```python
from build123d import *

# Parameters (mm, degrees)
SKETCH_2_R          = 1.5
CUT_EXTRUDE_1_DEPTH = 19.493242009


with BuildPart() as part:
    # 草图1 → 旋转1 (revolve)
    with BuildSketch(Plane.XY, mode=Mode.PRIVATE) as revolve_1_sk:
        Polygon((4, 0), (4, 15.5), (5, 15.5), (5, 5.5), (11, 5.5), (11, 2), (5, 2), (5, 0), align=None)
    revolve(revolve_1_sk.sketch.rotate(Axis((0, -4.166666667, 0), (0, 1, 0)), 90), axis=Axis((0, -4.166666667, 0), (0, 1, 0)))

    # 草图2 → 切除-拉伸1 (cut, through all)
    with BuildSketch(Plane(origin=(0, 5.5, 0), x_dir=(1, 0, 0), z_dir=(0, 1, 0))):
        with Locations(Location((0, 8, 0), (0, 0, 270))):
            Circle(SKETCH_2_R)
        with Locations(Location((8, 0, 0), (0, 0, 270))):
            Circle(SKETCH_2_R)
        with Locations(Location((0, -8, 0), (0, 0, 270))):
            Circle(SKETCH_2_R)
        with Locations(Location((-8, 0, 0), (0, 0, 270))):
            Circle(SKETCH_2_R)
    extrude(amount=-CUT_EXTRUDE_1_DEPTH, mode=Mode.SUBTRACT)


solid = part.part
```
Geometry: final body of the model. Coordinates: model frame, mm. A direction names the side the tool comes from. Round coordinates to 2 decimals unless told otherwise and drop trailing zeros. Write each loop counter-clockwise with the first axis right and the second up, starting at its lowest first coordinate (ties: lowest second). Pieces come first, ordered by that corner, then holes. Notation, with made-up numbers: (64, 73.25) -> (90, 73.25) arc R19 ccw to (90, 90.25) -> close; hole circle Ø10 at (13, -16). An arc over 180 degrees is marked (long way). Use CSV: the item, a comma, the result in double quotes. Start each with the question number.
Q1. Pull-direction query (X, two-part tool) for faces 4 (the face through (2, 5.5, 5)), 5 (the face through (0.07, 3.77, -9.5)), 6 (the face through (10.74, 3.73, 2.38)); classes: pulls with the +X half, pulls with the -X half, needs draft (parallel to the pull), parting line crosses it, or undercut.
Q2. Section C-C (y = 4.5). Return loops of the section in (x, z), plus the area to 3 significant figures.
Q3. Section B-B (x = 0). Return loops of the section in (y, z).
Q4. First-contact query: pin 1 Ø1.8 at (x, z) = (0, -8) entering from -Y; pin 2 Ø5 at (x, z) = (-8, 0) entering from +Y; pin 3 Ø6 at (y, z) = (5, 4) entering from +X; pin 4 Ø4 at (x, z) = (8, -5) entering from -Y. Flat tips, straight axial feed; report the tip coordinate or a pass-through.
Q5. Reachability of faces 1 (the face through (5, 2, -2)), 2 (the face through (6.536, 3.774, -0.325)), 3 (the face through (0, 10, 5)) from +Z, -Z, +X, -X, +Y, -Y: full face, straight path, thin tool, end or side. Return the list, or none.
Q6. Section A-A (z = 0). Return loops of the section in (x, y), plus the area to 3 significant figures.
Q7. Section D-D (z = -7.5). Return loops of the section in (x, y), plus the area to 3 significant figures.
Q8. Line query: L1, parallel to X at y = 3.1, z = 0; L2, parallel to Y at x = 2.75, z = 4.5; L3, parallel to Z at x = -3, y = 4. Output: solid intervals per line, ascending.
Result sheet:
1,face 4,"needs draft"
1,face 5,"undercut"
1,face 6,"parting line crosses it"
2,outline,"circle Ø22 at (0, 0); hole circle Ø3 at (-8, 0); hole circle Ø8 at (0, 0); hole circle Ø3 at (0, -8); hole circle Ø3 at (0, 8); hole circle Ø3 at (8, 0)"
2,area,"302 mm²"
3,outline,"(0, -5) -> (2, -5) -> (2, -6.5) -> (5.5, -6.5) -> (5.5, -5) -> (15.5, -5) -> (15.5, -4) -> (0, -4) -> close; (0, 4) -> (15.5, 4) -> (15.5, 5) -> (5.5, 5) -> (5.5, 6.5) -> (2, 6.5) -> (2, 5) -> (0, 5) -> close; (2, -11) -> (5.5, -11) -> (5.5, -9.5) -> (2, -9.5) -> close; (2, 9.5) -> (5.5, 9.5) -> (5.5, 11) -> (2, 11) -> close"
4,pin 1,"through"
4,pin 2,"y = 5.5"
4,pin 3,"x = 10.95"
4,pin 4,"y = 2"
5,face 1,"-Y"
5,face 2,"+Y, -Y"
5,face 3,"+Y"
6,outline,"(-11, 2) -> (-9.5, 2) -> (-9.5, 5.5) -> (-11, 5.5) -> close; (-6.5, 2) -> (-5, 2) -> (-5, 0) -> (-4, 0) -> (-4, 15.5) -> (-5, 15.5) -> (-5, 5.5) -> (-6.5, 5.5) -> close; (4, 0) -> (5, 0) -> (5, 2) -> (6.5, 2) -> (6.5, 5.5) -> (5, 5.5) -> (5, 15.5) -> (4, 15.5) -> close; (9.5, 2) -> (11, 2) -> (11, 5.5) -> (9.5, 5.5) -> close"
6,area,"52.0 mm²"
7,outline,"(-8.05, 2) -> (-1.41, 2) -> (-1.41, 5.5) -> (-8.05, 5.5) -> close; (1.41, 2) -> (8.05, 2) -> (8.05, 5.5) -> (1.41, 5.5) -> close"
7,area,"46.4 mm²"
8,L1,"-11 to -9.5, -6.5 to -4, 4 to 6.5, 9.5 to 11"
8,L2,"2 to 5.5"
8,L3,"-10.58 to -2.65, 2.65 to 10.58"
